Source: three-view drawing plus pictorial views. Frame: mm from the lowest corner of the part. A direction names the side the tool comes from. Give positions to 0.01 mm unless a question says otherwise; leave off trailing zeros. Loops run counter-clockwise (first coordinate to the right, second up) from the corner with the lowest first, then second, coordinate; pieces in that order, holes last.
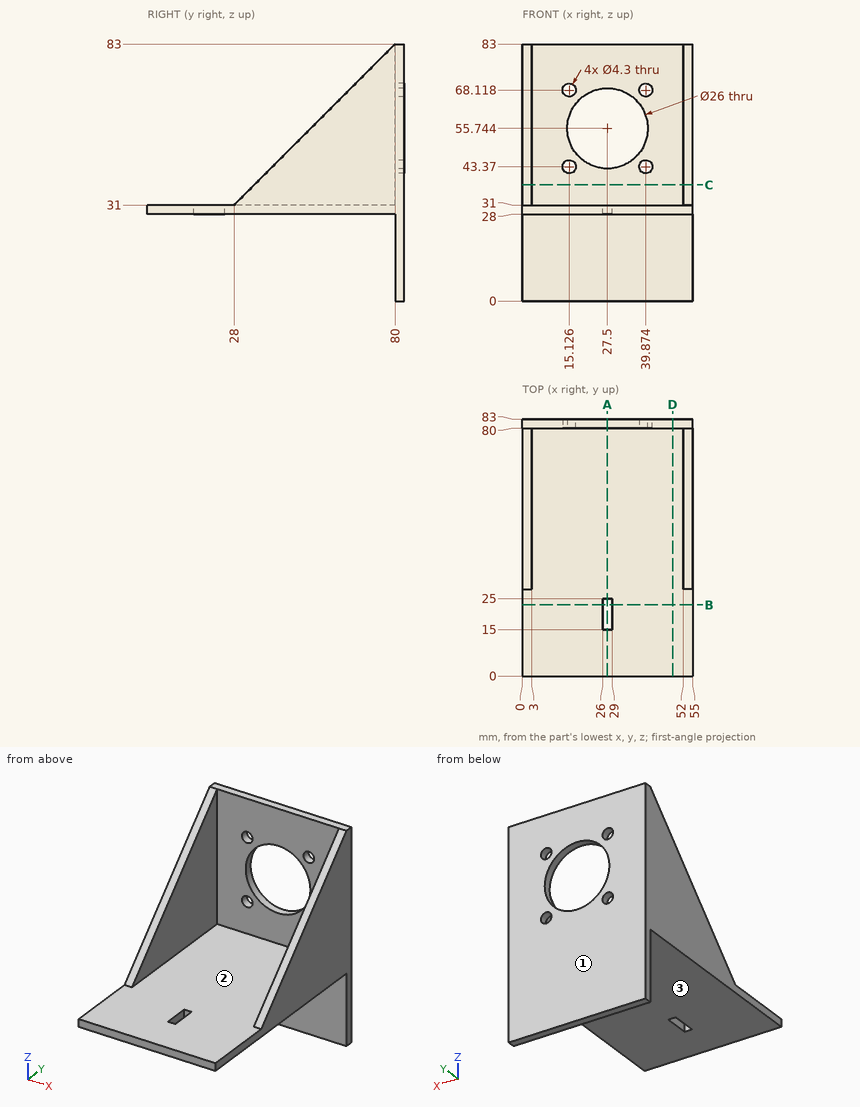
(1) Ray query, probe 1 along X at (y, z) = (53.5, 52); probe 2 along Y at (x, z) = (22, 22); probe 3 along Z at (x, y) = (7.5, 41). Return the intervals inside material, ascending.
Values follow:
probe 1: x = 0 to 3, 52 to 55
probe 2: y = 80 to 83
probe 3: z = 28 to 31
(2) Cut plane D-D (x = 48.5). Return the cut outline in (y, z), and give its area (3 significant figures).
Values follow:
outline: (0, 28) - (80, 28) - (80, 0) - (83, 0) - (83, 83) - (80, 83) - (80, 31) - (0, 31) - close
area: 489 mm2
(3) Reachability of the marked faces 1, 2 and 3 from +Z, -Z, +X, -X, +Y, -Y: full face, straight path, thin tool, end or side. Return the list, or none.
Values follow:
face 1: +Z, -Z, +X, -X, +Y
face 2: +Z, -Y
face 3: -Z, +X, -X, -Y
(4) Pin query (flat end, axial travel): pin 1 Ø5 at (x, y) = (31, 21) entering from +Z; pin 2 Ø2 at (x, y) = (24, 15.5) entering from -Z; pin 3 Ø2 at (y, z) = (74.5, 68) entering from -X; pin 4 Ø22.5 at (x, z) = (33.5, 10.5) entering from -Y. Return the tip coordinate at first contact, or that it passes through.
Values follow:
pin 1: stops at z = 31
pin 2: stops at z = 28
pin 3: stops at x = 0
pin 4: stops at y = 80
(5) Cut plane B-B (y = 23). Return the cut outline in (x, z).
Values follow:
outline: (0, 28) - (26, 28) - (26, 31) - (0, 31) - close; (29, 28) - (55, 28) - (55, 31) - (29, 31) - close
(6) Cut plane C-C (z = 37.5). Return the cut outline in (x, y).
Values follow:
outline: (0, 34.5) - (3, 34.5) - (3, 80) - (52, 80) - (52, 34.5) - (55, 34.5) - (55, 83) - (0, 83) - close
(7) Cut plane A-A (x = 27.5). Return the cut outline in (y, z).
Values follow:
outline: (0, 28) - (15, 28) - (15, 31) - (0, 31) - close; (25, 28) - (80, 28) - (80, 0) - (83, 0) - (83, 42.74) - (80, 42.74) - (80, 31) - (25, 31) - close; (80, 68.74) - (83, 68.74) - (83, 83) - (80, 83) - close
